For this review, take the finished solid that the model builds, in its own axes (mm). A direction names the side the tool comes from. Coordinates: 2 decimals unless noted, no trailing zeros. Order: outer loops, then holes, each group sorted by start corner. A loop starts at its lowest first (then second) coordinate and runs counter-clockwise, first axis right, second up.
from build123d import *

# Parameters (mm, degrees)
BOSS_EXTRUDE1_DEPTH = 8
CHAMFER5_SIZE       = 5
FILLET1_R           = 2.5
SKETCH2_R           = 1.5
CUT_EXTRUDE1_DEPTH  = 63.819184968
SKETCH3_R           = 1.8
CUT_EXTRUDE2_DEPTH  = 60.634302209
SKETCH5_W           = 8.5
SKETCH5_H           = 8
CUT_EXTRUDE3_DEPTH  = 15
CUT_EXTRUDE5_DEPTH  = 15


with BuildPart() as part:
    # Sketch1 → Boss-Extrude1 (new, symmetric)
    with BuildSketch(Plane.XY):
        Polygon((-50, 0), (-33, 0), (-33, 30), (33, 30), (33, 0), (50, 0), (50, 3), (41.5, 3), (41.5, 34.5), (-41.5, 34.5), (-41.5, 3), (-50, 3), align=None)
    extrude(amount=BOSS_EXTRUDE1_DEPTH, both=True)

    # Chamfer5
    chamfer5_edges = [part.edges().sort_by_distance(p)[0] for p in [
        (-41.5, 34.5, 0),
        (41.5, 34.5, 0),
        (33, 0, 0),
        (-33, 0, 0),
    ]]
    chamfer(chamfer5_edges, length=CHAMFER5_SIZE)

    # Fillet1
    fillet1_edges = [part.edges().sort_by_distance(p)[0] for p in [
        (-41.5, 3, 0),
        (41.5, 3, 0),
    ]]
    fillet(fillet1_edges, radius=FILLET1_R)

    # Sketch2 → Cut-Extrude1 (cut, through all)
    with BuildSketch(Plane.XY.offset(8)):
        with Locations((38, 23.5)):
            Circle(SKETCH2_R)
        with Locations((38, 6.5)):
            Circle(SKETCH2_R)
    cut_extrude1 = extrude(amount=-CUT_EXTRUDE1_DEPTH, mode=Mode.SUBTRACT)

    # Mirror1: Cut-Extrude1 across plane
    add(cut_extrude1.mirror(Plane(origin=(0, 0, 0), x_dir=(0, 0, 1), z_dir=(1, 0, 0))), mode=Mode.SUBTRACT)

    # Sketch3 → Cut-Extrude2 (cut, through all)
    with BuildSketch(Plane(origin=(0, 3, 0), x_dir=(1, 0, 0), z_dir=(0, 1, 0))):
        with Locations(Location((46, 4, 0), (0, 0, 270))):
            Circle(SKETCH3_R)
        with Locations(Location((46, -4, 0), (0, 0, 270))):
            Circle(SKETCH3_R)
        with Locations(Location((-46, 4, 0), (0, 0, 270))):
            Circle(SKETCH3_R)
        with Locations(Location((-46, -4, 0), (0, 0, 270))):
            Circle(SKETCH3_R)
    extrude(amount=-CUT_EXTRUDE2_DEPTH, mode=Mode.SUBTRACT)

    # Sketch5 → Cut-Extrude3 (cut)
    with BuildSketch(Plane(origin=(0, 34.5, 0), x_dir=(1, 0, 0), z_dir=(0, 1, 0))):
        with Locations((37.25, 0)):
            Rectangle(SKETCH5_W, SKETCH5_H)
        with Locations((-37.25, 0)):
            Rectangle(SKETCH5_W, SKETCH5_H)
    extrude(amount=-CUT_EXTRUDE3_DEPTH, mode=Mode.SUBTRACT)

    # Sketch7 → Cut-Extrude5 (cut)
    with BuildSketch(Plane(origin=(0, 34.5, 0), x_dir=(1, 0, 0), z_dir=(0, 1, 0))):
        with BuildLine():
            Line((33, 4), (33, -4))
            ThreePointArc((33, -4), (29, 0), (33, 4))
        make_face()
        with BuildLine():
            Line((-33, 4), (-33, -4))
            ThreePointArc((-33, -4), (-29, 0), (-33, 4))
        make_face()
    extrude(amount=-CUT_EXTRUDE5_DEPTH, mode=Mode.SUBTRACT)


solid = part.part
1. Take a section at B-B, the plane z = -1. Give the boundary of the cut face in (x, y), plus the area to 3 significant figures.
Answer below:
outline: (-50, 0) - (-38, 0) - (-33, 5) - (-33, 19.5) - (-41.5, 19.5) - (-41.5, 5.5) arc R2.5 cw to (-44, 3) - (-50, 3) - close; (-29.13, 30) - (29.13, 30) - (29.13, 34.5) - (-29.13, 34.5) - close; (33, 5) - (38, 0) - (50, 0) - (50, 3) - (44, 3) arc R2.5 cw to (41.5, 5.5) - (41.5, 19.5) - (33, 19.5) - close; hole circle Ø3 at (-38, 6.5); hole circle Ø3 at (38, 6.5)
area: 608 mm2
2. To check wall thickness, follow L1, parallel to Y at x = 38, z = 5.45; L2, parallel to X at y = 19.5, z = 5.25; L3, parallel to Z at x = -37, y = 28.5. State the ranges of each line that lie inside material, in increasing order.
Answer below:
L1: y = 0 to 5, 8 to 22, 25 to 33
L2: x = -41.5 to -33, 33 to 41.5
L3: z = -8 to -4, 4 to 8
3. Take a section at D-D, the plane y = 32. Give the boundary of the cut face in (x, z).
Answer below:
outline: (-39, -8) - (39, -8) - (39, -4) - (33, -4) arc R4 cw to (33, 4) - (39, 4) - (39, 8) - (-39, 8) - (-39, 4) - (-33, 4) arc R4 cw to (-33, -4) - (-39, -4) - close
4. Take a section at C-C, the plane y = 6.5. Give the boundary of the cut face in (x, z), plus the area to 3 significant figures.
Answer below:
outline: (-41.5, -8) - (-39.5, -8) - (-39.5, 8) - (-41.5, 8) - close; (-36.5, -8) - (-33, -8) - (-33, 8) - (-36.5, 8) - close; (33, -8) - (36.5, -8) - (36.5, 8) - (33, 8) - close; (39.5, -8) - (41.5, -8) - (41.5, 8) - (39.5, 8) - close
area: 176 mm2
5. Machinability: for faces 4 (the face through (37, 19.5, 0)), 5 (the face through (-47, 3, 0)), 6 (the face through (41.5, 15, 0)), which of the approach directions +Z, -Z, +X, -X, +Y, -Y give a long, thin tool a straight path to every point of the face, cutting with its end or side? Answer none if there is none.
Answer below:
face 4: +X, -X, +Y
face 5: +Z, -Z, -X, +Y
face 6: +Z, -Z, +X, +Y
6. Clearance check with flat-ended pins moving along their axes: pin 1 Ø5 at (y, z) = (11.5, 3) entering from +X; pin 2 Ø3 at (x, z) = (48, -2) entering from +Y; pin 3 Ø5 at (x, z) = (8.5, 2.5) entering from -Y. State where each tip first meets the part, or that it passes through.
Answer below:
pin 1: stops at x = 41.5
pin 2: stops at y = 3
pin 3: stops at y = 30
7. Take a section at A-A, the plane y = 23.5. Give the number of separate pieces and of enclosed holes in the cut face, plus the area to 3 significant figures.
Answer below:
separate pieces: 8
enclosed holes: 0
area: 88.0 mm2
8. The part is to be moulded in two halves that separate along Y. For faces 1 (the face through (47.785, 1.521, 3.766)), 2 (the face through (47, 3, 0)), 3 (the face through (-36.8, 5.6, 0.1)), say which applies: +Y half, -Y half, draft (parallel to the pull), parting line (faces both ways), or undercut.
Answer below:
face 1: draft
face 2: +Y half
face 3: undercut
